Source: CAD feature listing. Evaluate the final solid. Frame: model axes, mm. A direction names the side the tool comes from. Give positions to 0.01 mm unless a question says otherwise; leave off trailing zeros. Order: outer loops, then holes, each group sorted by start corner. A loop starts at its lowest first (then second) coordinate and runs counter-clockwise, first axis right, second up.
from build123d import *

# Parameters (mm, degrees)
F2_R = 10


with BuildPart() as f1:
    # F0 (on Right) → F1 (revolve)
    with BuildSketch(Plane.YZ):
        Polygon((-50, 15), (-48.5, 15), (-48.5, 59.310098), (-13.5, 89.310098), (-13.5, 122.471504), (-1.1, 122.471504), (-1.1, 127.54637), (-1.5, 127.54637), (-1.5, 128.5), (-3.1, 128.5), (-3.1, 130), (-15, 130), (-15, 90), (-50, 60), align=None)
    revolve(axis=Axis((0, 0, 8.976309), (0, 0, 1)))

    # F2
    f2_edges = [f1.edges().sort_by_distance(p)[0] for p in [
        (0, 50, 60),
    ]]
    fillet(f2_edges, radius=F2_R)


solid = f1.part
(1) Line query: line 1 along Y through (x, z) = (0.5, 23); line 2 along X through (y, z) = (0, 129.35). Output: solid intervals per line, ascending.
(2) Section B-B, the plane z = 110. Return loops of the section in (x, y).
(3) Draft query along Y for faces 4 (the cylindrical face through (-43.028, -22.38, 37.465)), 5 (the flat face through (4, 0, 130)), 6 (the cylindrical face through (0.66, 14.985, 109.72)). Return one class per face: +Y half, -Y half, draft (parallel to the pull), parting line (faces both ways), or undercut.
(4) Section A-A, the plane z = 37. Return loops of the section in (x, y), plus the area to 3 significant figures.
(5) Pin query (flat end, axial travel): pin 1 Ø10 at (y, z) = (6, 35) entering from +X; pin 2 Ø10 at (y, z) = (23, 79) entering from +X; pin 3 Ø1.5 at (y, z) = (-9.5, 46) entering from -X; pin 4 Ø1.8 at (x, y) = (0, 0) entering from -Z. Return the tip coordinate at first contact, or that it passes through.
(6) Access query for faces 1 (the flat face through (41, 26.2, 15)), 2 (the flat face through (0, -3, 122.472)), 3 (the cylindrical face through (-2.75, -1.43, 129.26)). Directions: +Z, -Z, +X, -X, +Y, -Y. A direction counts if a zero-diameter tool reaches every point of the face in a straight line with its end or side. Return the directions, or none.
Checks:
1. line 1: y = -50 to -48.5, 48.5 to 50
1. line 2: x = -15 to -3.1, 3.1 to 15
2. outline: circle Ø30 at (0, 0); hole circle Ø27 at (0, 0)
3. face 4: undercut
3. face 5: draft
3. face 6: parting line
4. outline: circle Ø100 at (0, 0); hole circle Ø97 at (0, 0)
4. area: 464 mm2
5. pin 1: stops at x = 49.99
5. pin 2: stops at x = 25.72
5. pin 3: stops at x = -49.23
5. pin 4: passes through
6. face 1: -Z, +X, -X, +Y, -Y
6. face 2: -Z
6. face 3: +Z
